For this review, take the finished solid that the model builds, in its own axes (mm). A direction names the side the tool comes from. Round coordinates to 2 decimals unless told otherwise and drop trailing zeros. Order: outer loops, then holes, each group sorted by start corner. A loop starts at its lowest first (then second) coordinate and runs counter-clockwise, first axis right, second up. Notation, with made-up numbers: (7.25, 35.25) -> (65.25, 35.25) arc R20 cw to (65.25, 68.25) -> close; hole circle Ø4 at (17.5, 89). An arc over 180 degrees is marked (long way). Use a Markdown table: item, result. Add a question column.
1) Machinability: for faces 4 (the face through (-2, 2, 1)), 5 (the face through (2.1, 2.14, 3.52)), 6 (the face through (-2.1, 4.49, 4.14)), which of the approach directions +Z, -Z, +X, -X, +Y, -Y give a long, thin tool a straight path to every point of the face, cutting with its end or side? Answer none if there is none.
2) Consider section D-D (x = -1.25). State the section outline as (y, z) points, plus the area to 3 significant figures.
3) Consider section C-C (z = 4.5). State the section outline as (x, y) points.
4) Wall thickness on line 1 along X through (y, z) = (0, 0.6); line 2 along X through (y, z) = (3.5, 3.25): over which ranges is each line inside the solid? List them lowest first. Write a range as [from, to].
5) Consider section B-B (x = 0.5). State the section outline as (y, z) points, plus the area to 3 significant figures.
6) Consider section A-A (z = 0.9). State the section outline as (x, y) points, plus the area to 3 significant figures.
7) Draft analysis for pull direction X (two halves, no side actions). For faces 1 (the face through (5, 2, 2)), 2 (the face through (1, 1, 2)), 3 (the face through (0, -1, 1)), state which applies: pulls with the +X half, pulls with the -X half, needs draft (parallel to the pull), parting line crosses it, or undercut.
8) Clearance check with flat-ended pins moving along their axes: P1, Ø0.5, axis at y = 3.5, z = 4, coming from the -X side; P2, Ø1.5, axis at x = 1, y = 0, coming from the +Z side; P3, Ø1.6, axis at y = 1.5, z = 1, coming from the -X side. State where each tip first meets the part, or that it passes through.
```python
from build123d import *

# Parameters (mm, degrees)
SKETCH1_R           = 1
BOSS_EXTRUDE1_DEPTH = 5
SKETCH2_OUTSIDE_W   = 12.35
SKETCH2_OUTSIDE_H   = 11.35
CUT_EXTRUDE1_DEPTH  = 3
CUT_EXTRUDE2_DEPTH  = 3
CUT_EXTRUDE3_DEPTH  = 3


with BuildPart() as part:
    # Sketch1 → Boss-Extrude1 (new body)
    with BuildSketch(Plane.XY):
        with BuildLine():
            Line((-2, 0), (-2, 4))
            Line((-2, 4), (-3, 4))
            Line((-3, 4), (-3, 5))
            Line((-3, 5), (5, 5))
            Line((5, 5), (5, -2))
            Line((5, -2), (0, -2))
            ThreePointArc((0, -2), (-1.414213562, -1.414213562), (-2, 0))
        make_face()
        Circle(SKETCH1_R, mode=Mode.SUBTRACT)
    extrude(amount=BOSS_EXTRUDE1_DEPTH)

    # Sketch2 outside → Cut-Extrude1 (cut)
    with BuildSketch(Plane.XY.offset(5)):
        with Locations((1, 1.5)):
            Rectangle(SKETCH2_OUTSIDE_W, SKETCH2_OUTSIDE_H)
        with BuildLine():
            Line((5, -2), (5, 5))
            Line((5, 5), (-3, 5))
            Line((-3, 5), (-3, 4))
            Line((-3, 4), (-2, 4))
            Line((-2, 4), (0, 4))
            Line((0, 4), (0, 3))
            ThreePointArc((0, 3), (2.121320344, 2.121320344), (3, 0))
            Line((3, 0), (3, -2))
            Line((3, -2), (5, -2))
        make_face(mode=Mode.SUBTRACT)
    extrude(amount=-CUT_EXTRUDE1_DEPTH, mode=Mode.SUBTRACT)

    # Sketch3 → Cut-Extrude2 (cut)
    with BuildSketch(Plane.XZ.offset(-4)):
        with BuildLine():
            Line((-3, 2), (-3, 5))
            Line((-3, 5), (0, 5))
            ThreePointArc((0, 5), (-2.121320344, 4.121320344), (-3, 2))
        make_face()
    extrude(amount=-CUT_EXTRUDE2_DEPTH, mode=Mode.SUBTRACT)

    # Sketch4 → Cut-Extrude3 (cut, through all)
    with BuildSketch(Plane.ZY.offset(-3)):
        Polygon((5, 0), (3, -2), (5, -2), align=None)
    extrude(amount=-CUT_EXTRUDE3_DEPTH, mode=Mode.SUBTRACT)


solid = part.part
```
Results list:
| question | item | result |
|---|---|---|
| 1 | face 4 | +Z, -Z, -X, -Y |
| 1 | face 5 | +Z, -X, -Y |
| 1 | face 6 | +Z, -X, +Y, -Y |
| 2 | outline | (-1.56, 0) -> (5, 0) -> (5, 4.73) -> (4, 4.73) -> (4, 2) -> (-1.56, 2) -> close |
| 2 | area | 15.8 mm2 |
| 3 | outline | (-1.66, 4) -> (0, 4) -> (0, 3) arc R3 cw to (3, 0) -> (3, -0.5) -> (5, -0.5) -> (5, 5) -> (-1.66, 5) -> close |
| 4 | line 1 | [-2, -1], [1, 5] |
| 4 | line 2 | [0, 5] |
| 5 | outline | (-2, 0) -> (-0.87, 0) -> (-0.87, 2) -> (-2, 2) -> close; (0.87, 0) -> (5, 0) -> (5, 5) -> (2.96, 5) -> (2.96, 2) -> (0.87, 2) -> close |
| 5 | area | 16.7 mm2 |
| 6 | outline | (-3, 4) -> (-2, 4) -> (-2, 0) arc R2 ccw to (0, -2) -> (5, -2) -> (5, 5) -> (-3, 5) -> close; hole circle Ø2 at (0, 0) |
| 6 | area | 46.0 mm2 |
| 7 | face 1 | pulls with the +X half |
| 7 | face 2 | needs draft |
| 7 | face 3 | undercut |
| 8 | P1 | x = 0 |
| 8 | P2 | z = 2 |
| 8 | P3 | x = -2 |
